CAD build for the part. Positions are in the model's coordinates, mm. Give positions to 0.01 mm unless a question says otherwise; leave off trailing zeros. Loops run counter-clockwise (first coordinate to the right, second up) from the corner with the lowest first, then second, coordinate; pieces in that order, holes last. Notation, with made-up numbers: (58, 87) - (94, 87) arc R19 cw to (94, 96) - close; hole circle Ø3 at (51.5, 39). An arc over 180 degrees is marked (long way). Return JSON: item names as keys, results as strings.
from build123d import *

# Parameters (mm, degrees)
PAD_DEPTH    = 2700
SKETCH_R     = 10
PAD001_DEPTH = 80
SKETCH002_R  = 10
PAD002_DEPTH = 80


with BuildPart() as part:
    # Sketch001 → Pad (new body)
    with BuildSketch(Plane.YZ):
        Polygon((0, 0), (0, -10), (2, -10), (2, -30), (0, -30), (0, -65), (2, -65), (2, -75), (0, -75), (0, -110), (2, -110), (2, -130), (0, -130), (0, -140), (50, -140), (50, -130), (48, -130), (48, -110), (50, -110), (50, -75), (48, -75), (48, -65), (50, -65), (50, -30), (48, -30), (48, -10), (50, -10), (50, 0), align=None)
    extrude(amount=PAD_DEPTH)

    # Sketch (on Face29 of Pad) → Pad001 (join)
    with BuildSketch(Plane(origin=(0, 0, 0), x_dir=(0, 1, 0), z_dir=(-1, 0, 0))):
        with Locations((25, 100)):
            Circle(SKETCH_R)
        with Locations((25, 40)):
            Circle(SKETCH_R)
    extrude(amount=PAD001_DEPTH)

    # Sketch002 (on Face5 of Pad001) → Pad002 (join)
    with BuildSketch(Plane.YZ.offset(2700)):
        with Locations((25, -40)):
            Circle(SKETCH002_R)
        with Locations((25, -100)):
            Circle(SKETCH002_R)
    extrude(amount=PAD002_DEPTH)


solid = part.part
1. Cut at B-B, the plane x = 435.5. Write the cut outline in (y, z), plus the area to 3 significant figures.
Values follow:
{"outline": "(0, -140) - (50, -140) - (50, -130) - (48, -130) - (48, -110) - (50, -110) - (50, -75) - (48, -75) - (48, -65) - (50, -65) - (50, -30) - (48, -30) - (48, -10) - (50, -10) - (50, 0) - (0, 0) - (0, -10) - (2, -10) - (2, -30) - (0, -30) - (0, -65) - (2, -65) - (2, -75) - (0, -75) - (0, -110) - (2, -110) - (2, -130) - (0, -130) - close", "area": "6,800 mm²"}
2. Drill centre lines: probe 1 along X at (y, z) = (37.5, -125.5); probe 2 along Y at (x, z) = (730, -117.5). Where is each one in solid material? Low to high.
Values follow:
{"probe 1": "x = 0 to 2700", "probe 2": "y = 2 to 48"}
3. Cut at A-A, the plane y = 25. Write the cut outline in (x, z).
Values follow:
{"outline": "(-80, -110) - (0, -110) - (0, -140) - (2700, -140) - (2700, -110) - (2780, -110) - (2780, -90) - (2700, -90) - (2700, -50) - (2780, -50) - (2780, -30) - (2700, -30) - (2700, 0) - (0, 0) - (0, -30) - (-80, -30) - (-80, -50) - (0, -50) - (0, -90) - (-80, -90) - close"}
4. Drop flat-ended pins along their axis: P1, Ø1.5, axis at y = 5, z = -75, coming from the -X side; P2, Ø10, axis at x = 2004.5, z = -124, coming from the -Y side; P3, Ø2, axis at y = 44, z = -37, coming from the +X side. Give the stop position or say it passes through.
Values follow:
{"P1": "stops at x = 0", "P2": "stops at y = 2", "P3": "stops at x = 2700"}
